Can you work these out from the model? Positions are in its coordinate system, mm. Face numbers are marked on the shaded views. Coordinates: 2 decimals unless noted, no trailing zeros. Loops run counter-clockwise (first coordinate to the right, second up) from the corner with the lowest first, then second, coordinate; pieces in that order, holes last.
```python
from build123d import *

# Parameters (mm, degrees)
SKETCH_1_R          = 2.1
EXTRUDE_4_DEPTH     = 0.8
SKETCH_2_R          = 2.25
SKETCH_2_R_2        = 1
EXTRUDE_5_DEPTH     = 3
FILLET_1_R          = 0.5
SKETCH_3_W          = 6.892182162
SKETCH_3_H          = 5.392211784
SKETCH_3_R          = 2.25
CUT_EXTRUDE_1_DEPTH = 2


with BuildPart() as part:
    # Эскиз1 → Вытянуть4 (new body)
    with BuildSketch(Plane.XY):
        with BuildLine():
            Line((-0.65, 4.030380872), (4.098720888, 4.030380872))
            ThreePointArc((4.098720888, 4.030380872), (5.145271439, 2.513906235), (6.892973224, 1.930380872))
            Line((6.892973224, 1.930380872), (10.25, 1.930380872))
            Line((10.25, 1.930380872), (10.25, 0.180380872))
            Line((10.25, 0.180380872), (10.25, -2.069619128))
            Line((10.25, -2.069619128), (6.892973224, -2.069619128))
            ThreePointArc((6.892973224, -2.069619128), (5.145271439, -2.653144492), (4.098720888, -4.169619128))
            Line((4.098720888, -4.169619128), (-0.65, -4.169619128))
            ThreePointArc((-0.65, -4.169619128), (-4.75, -0.069619128), (-0.65, 4.030380872))
        make_face()
        with Locations((-0.65, -0.069619128)):
            Circle(SKETCH_1_R, mode=Mode.SUBTRACT)
    extrude(amount=EXTRUDE_4_DEPTH)

    # Эскиз2 → Вытянуть5 (add)
    with BuildSketch(Plane(origin=(10.25, 0, 0), x_dir=(0, 0, -1), z_dir=(1, 0, 0))):
        with Locations((-2.25, 0)):
            Circle(SKETCH_2_R)
        with Locations((-2.25, 0)):
            Circle(SKETCH_2_R_2, mode=Mode.SUBTRACT)
    extrude(amount=-EXTRUDE_5_DEPTH)

    # Скругление1
    fillet_1_edges = [part.edges().sort_by_distance(p)[0] for p in [
        (4.098720888, -4.169619128, 0.4),
        (4.098720888, 4.030380872, 0.4),
    ]]
    fillet(fillet_1_edges, radius=FILLET_1_R)

    # Эскиз3 → Вырез-Вытянуть1 (cut)
    with BuildSketch(Plane(origin=(10.25, 0, 0), x_dir=(0, 0, -1), z_dir=(1, 0, 0))):
        with Locations((-2.090078371, -0.255202745)):
            Rectangle(SKETCH_3_W, SKETCH_3_H)
        with Locations((-2.25, 0)):
            Circle(SKETCH_3_R, mode=Mode.SUBTRACT)
    extrude(amount=-CUT_EXTRUDE_1_DEPTH, mode=Mode.SUBTRACT)


solid = part.part
```
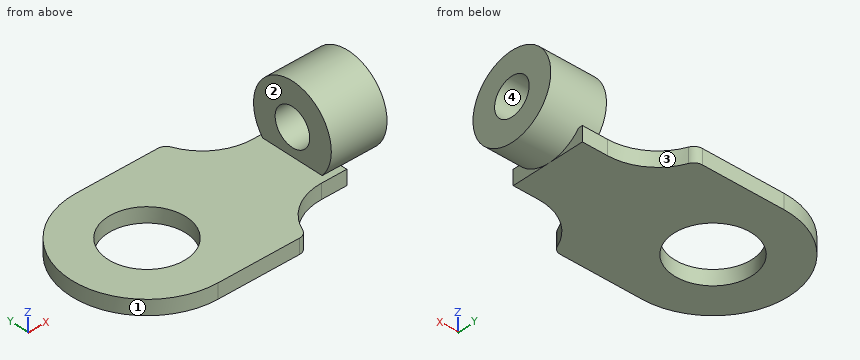
Item 1: I need wall thicknesses on line 1 along Y through (x, z) = (8.2, 2.25); line 2 along Y through (x, z) = (-0.65, 0.4); line 3 along Z through (x, y) = (4.75, 2). Which ranges of each line are inside material? Lowest first, please.
Results are:
line 1: y = -2.25 to -1, 1 to 2.25
line 2: y = -4.17 to -2.17, 2.03 to 4.03
line 3: z = 0 to 0.8
Item 2: Suppose I cut it at B-B, the plane x = 0.75. Please give me the cut outline in (y, z).
Results are:
outline: (-4.17, 0) - (-1.63, 0) - (-1.63, 0.8) - (-4.17, 0.8) - close; (1.5, 0) - (4.03, 0) - (4.03, 0.8) - (1.5, 0.8) - close
Item 3: I'm going to push flat-ended pins straight in: P1, Ø3, axis at x = 5, y = 2.5, coming from the +Z side; P2, Ø1.8, axis at y = 0, z = 2.25, coming from the +X side; P3, Ø2, axis at x = 5.5, z = 1.5, coming from the -Y side; P4, Ø1.8, axis at y = -0.5, z = 3, coming from the -X side. Where does each tip first touch, or does it pass through?
Results are:
P1: stops at z = 0.8
P2: passes through
P3: stops at y = -2.97
P4: stops at x = 7.25
Item 4: Suppose I cut it at C-C, the plane y = -0.75. Please give me the cut outline in (x, z).
Results are:
outline: (-4.69, 0) - (-2.64, 0) - (-2.64, 0.8) - (-4.69, 0.8) - close; (1.34, 0) - (8.25, 0) - (8.25, 0.13) - (10.25, 0.13) - (10.25, 1.59) - (7.25, 1.59) - (7.25, 0.8) - (1.34, 0.8) - close; (7.25, 2.91) - (10.25, 2.91) - (10.25, 4.37) - (7.25, 4.37) - close
Item 5: Suppose I cut it at A-A, the plane z = 2.25. Please give me the cut outline in (x, y).
Results are:
outline: (7.25, -2.25) - (10.25, -2.25) - (10.25, -1) - (7.25, -1) - close; (7.25, 1) - (10.25, 1) - (10.25, 2.25) - (7.25, 2.25) - close
Item 6: We'd pull the mould along Y, two halves only. Please class the marked faces 1, 2, 3 and 4: +Y half, -Y half, draft (parallel to the pull), parting line (faces both ways), or undercut.
Results are:
face 1: parting line
face 2: draft
face 3: +Y half
face 4: undercut
Item 7: Suppose I cut it at D-D, the plane y = 1.5. Please give me the cut outline in (x, z), plus the area to 3 significant figures.
Results are:
outline: (-4.44, 0) - (-2.05, 0) - (-2.05, 0.8) - (-4.44, 0.8) - close; (0.75, 0) - (8.25, 0) - (8.25, 0.57) - (10.25, 0.57) - (10.25, 3.93) - (7.25, 3.93) - (7.25, 0.8) - (0.75, 0.8) - close
area: 17.8 mm2
